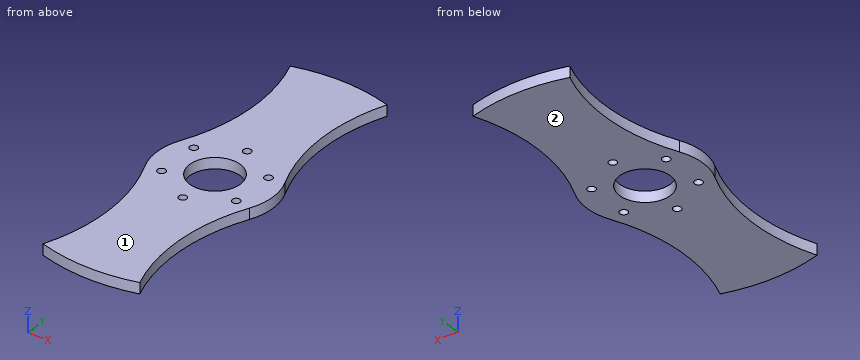
Autodesk Inventor part; units mm, degrees
ref_plane "YZ Plane" through (0, 0, 0) normal (1, 0, 0) x (0, 1, 0)
ref_plane "XZ Plane" through (0, 0, 0) normal (0, 1, 0) x (-1, 0, 0)
ref_plane "XY Plane" through (0, 0, 0) normal (0, 0, 1) x (1, 0, 0)
sketch "Sketch1" plane through (0, 0, 0) normal (0, 0, 1) x (1, 0, 0)
  circle A0 centre (0, 0) radius 11.1125
  line L0 (0, 0) -> (0, 19.05) construction
  circle A1 centre (0, 19.05) radius 1.7526
  circle A2 centre (-16.4978, 9.525) radius 1.7526
  circle A3 centre (-16.4978, -9.525) radius 1.7526
  circle A4 centre (0, -19.05) radius 1.7526
  circle A5 centre (16.4978, -9.525) radius 1.7526
  circle A6 centre (16.4978, 9.525) radius 1.7526
  circle A7 centre (0, 0) radius 76.2 construction
  line L1 (-15.875, -74.528) -> (15.875, -74.528) construction
  line L2 (15.875, -74.528) -> (15.875, 74.528) construction
  line L3 (15.875, 74.528) -> (-15.875, 74.528) construction
  line L4 (-15.875, 74.528) -> (-15.875, -74.528) construction
  line L5 (-15.875, -74.528) -> (15.875, 74.528) construction
  line L6 (15.875, -74.528) -> (-15.875, 74.528) construction
  line L7 (0, 76.2) -> (0, -76.2) construction
  line L8 (0, 0) -> (21.3699, 73.1421) construction
  circle A8 centre (0, 0) radius 66.675 construction
  circle A9 centre (0, 0) radius 25.4
  line L9 (21.3699, 73.1421) -> (17.8969, 64.2282) construction
  arc A10 (21.3699, 73.1421) -> (-21.3699, 73.1421) centre (0, 0) ccw
  line L10 (-15.875, 0) -> (15.875, 0) construction
  arc A11 (-21.3699, -73.1421) -> (21.3699, -73.1421) centre (0, 0) ccw
  arc A12 (21.3699, 73.1421) -> (23.1163, 10.5259) centre (96.4161, 43.9028) ccw
  arc A13 (-23.1163, 10.5259) -> (-21.3699, 73.1421) centre (-96.4161, 43.9028) ccw
  arc A14 (23.1163, -10.5259) -> (21.3699, -73.1421) centre (96.4161, -43.9028) ccw
  arc A15 (-21.3699, -73.1421) -> (-23.1163, -10.5259) centre (-96.4161, -43.9028) ccw
  point P0 (0, 74.528)
  point P1 (0, -66.675)
  point P2 (23.1163, -10.5259)
  point P3 (-23.1163, -10.5259)
  point P4 (-23.1163, 10.5259)
  dimension "d10" = 50.8
  dimension "d0" = 22.225
  dimension "d1" = 19.05
  dimension "d2" = 3.5052
  dimension "d5" = 360
  dimension "d7" = 152.4
  dimension "d8" = 31.75
  dimension "d9" = 9.525
  dimension "d11" = 5
extrude "Extrusion1" add sketch "Sketch1" along normal blind 4.7625
sketch "Sketch3" plane through (0, 0, 0) normal (0, 0, -1) x (-1, 0, 0)
  circle A0 centre (0, 0) radius 76.2 construction
  point P0 (21.3699, 73.1421)
  dimension "d25" = 152.4
properties part number "Blade (Bar)" material "Stainless Steel"
Design review of the part built by this model. Coordinates are the model's own, in mm. Face numbers are marked on the shaded views. Round coordinates to 2 decimals unless told otherwise and drop trailing zeros. Loops run counter-clockwise (first coordinate to the right, second up) from the corner with the lowest first, then second, coordinate; pieces in that order, holes last. Notation, with made-up numbers: M 72,87.25 L 87,87.25 A5 cw 87,93.25 Z; hole C 85.25,55.5 d11. An arc over 180 degrees is marked long. Answer as a JSON object with one key per item and string values.
Item 1: Wall thickness on L1, parallel to Y at x = -15, z = 3.65; L2, parallel to Y at x = -7, z = 3.9; L3, parallel to Y at x = 5, z = 1.4: over which ranges is each line inside the solid? List them lowest first. Write a range as from..to.
Answer sheet:
{"L1": "y = -74.71..-10.44, -8.61..8.61, 10.44..74.71", "L2": "y = -75.88..-8.63, 8.63..75.88", "L3": "y = -76.04..-9.92, 9.92..76.04"}
Item 2: We need section D-D on x = -8. Give the boundary of the cut face in (y, z), and give its area (3 significant figures).
Answer sheet:
{"outline": "M -75.78,0 L -7.71,0 L -7.71,4.76 L -75.78,4.76 Z; M 7.71,0 L 75.78,0 L 75.78,4.76 L 7.71,4.76 Z", "area": "648 mm^2"}
Item 3: The part is to be moulded in two halves that separate along Z. For the marked faces 1 and 2, say which applies: pulls with the +Z half, pulls with the -Z half, needs draft (parallel to the pull), parting line crosses it, or undercut.
Answer sheet:
{"face 1": "pulls with the +Z half", "face 2": "pulls with the -Z half"}
Item 4: We need section C-C on z = 1.4. State how many separate pieces and enclosed holes the cut face has, and give its area (3 significant figures).
Answer sheet:
{"separate pieces": "1", "enclosed holes": "7", "area": "5,270 mm^2"}
Item 5: Clearance check with flat-ended pins moving along their axes: P1, Ø2, axis at x = -16, z = 0.5, coming from the +Y side; P2, Ø1, axis at x = 12, z = 2.5, coming from the +Y side; P3, Ø2, axis at x = 4.5, z = 2.5, coming from the -Y side. State where each tip first meets the part, or that it passes through.
Answer sheet:
{"P1": "stops at y = 74.71", "P2": "stops at y = 75.33", "P3": "stops at y = -76.12"}
Item 6: We need section B-B on y = 0. Give the boundary of the cut face in (x, z).
Answer sheet:
{"outline": "M -25.4,0 L -11.11,0 L -11.11,4.76 L -25.4,4.76 Z; M 11.11,0 L 25.4,0 L 25.4,4.76 L 11.11,4.76 Z"}
Item 7: We need section A-A on x = 0. Give the boundary of the cut face in (y, z).
Answer sheet:
{"outline": "M -76.2,0 L -20.8,0 L -20.8,4.76 L -76.2,4.76 Z; M -17.3,0 L -11.11,0 L -11.11,4.76 L -17.3,4.76 Z; M 11.11,0 L 17.3,0 L 17.3,4.76 L 11.11,4.76 Z; M 20.8,0 L 76.2,0 L 76.2,4.76 L 20.8,4.76 Z"}
